Here's how the part is built. I have some questions about the finished solid (model axes, mm). Give positions to 0.01 mm unless a question says otherwise; leave off trailing zeros. Loops run counter-clockwise (first coordinate to the right, second up) from the corner with the lowest first, then second, coordinate; pieces in that order, holes last.
Q1. If we section it at A-A (z = 0): Please give me the cut outline in (x, y).
Q2. If we section it at B-B (x = -1.25): Please give me the cut outline in (y, z).
Q3. If we section it at D-D (z = 4.5): Please give me the cut outline in (x, y), plus the area to 3 significant figures.
Q4. I need wall thicknesses on line 1 (Y direction, x = -11.4, z = 0); line 2 (X direction, y = 6.25, z = -0.5); line 3 (X direction, y = 0.25, z = 9). Which ranges of each line are inside material? Lowest first, please.
Q5. We'd pull the mould along Z, two halves only. Please class faces 1 (the face through (-11.221, 9.541, 2.973)), 2 (the face through (-16.7, 0, 0)), 3 (the face through (-11.22, -9.75, 5.09)), 4 (the face through (-6.26, 0.54, 12.19)): +Z half, -Z half, draft (parallel to the pull), parting line (faces both ways), or undercut.
Q6. Will these pins go through, and if not, where does the flat tip stop? P1, Ø2, axis at x = -5, z = 2.5, coming from the -Y side; P2, Ø10, axis at x = -8, y = 8.5, coming from the +Z side; P3, Ø1.2, axis at y = 8.5, z = 5.5, coming from the -X side.
Q7. If we section it at C-C (z = -4.5): Please give me the cut outline in (x, y), plus the area to 3 significant figures.
from build123d import *

# Parameters (mm, degrees)
CUT_EXTRUDE_1_DEPTH = 3
SKETCH_4_R          = 0.75
CUT_EXTRUDE_2_DEPTH = 3
SKETCH_6_R          = 0.65
CUT_EXTRUDE_3_DEPTH = 3


with BuildPart() as part:
    # 草图1 → 旋转1 (revolve)
    with BuildSketch(Plane(origin=(0, 0, 0), x_dir=(1, 0, 0), z_dir=(0, 1, 0))):
        Polygon((0, 0), (-16.7, 0), (-16.7, 3), (-12.7, 3), (-12.7, 12.2), (0, 12.2), align=None)
    revolve(axis=Axis((-159.613189405, 0, 0), (1, 0, 0)))

    # 草图3 → 切除-拉伸1 (cut)
    with BuildSketch(Plane.ZY.offset(12.7)):
        with BuildLine():
            ThreePointArc((-8.667998766, 2.421940832), (-8.99040601, 0.415451281), (-8.854419452, -1.612220883))
            ThreePointArc((-8.854419452, -1.612220883), (-9.764043418, -2.198869939), (-10.822068219, -1.97049219))
            ThreePointArc((-10.822068219, -1.97049219), (-10.988274013, 0.507773788), (-10.594220714, 2.960149905))
            ThreePointArc((-10.594220714, 2.960149905), (-9.519642991, 3.089978996), (-8.667998766, 2.421940832))
        make_face()
        with BuildLine():
            ThreePointArc((6.43146167, 6.295736716), (4.854994369, 7.578194355), (3.030985485, 8.474262622))
            ThreePointArc((3.030985485, 8.474262622), (2.977744482, 9.555344613), (3.704537815, 10.357432094))
            ThreePointArc((3.704537815, 10.357432094), (5.933882006, 9.262237545), (7.860675374, 7.694789319))
            ThreePointArc((7.860675374, 7.694789319), (7.435821803, 6.699263167), (6.43146167, 6.295736716))
        make_face()
        with BuildLine():
            ThreePointArc((2.236537096, -8.717677547), (4.135411642, -7.993645636), (5.823433967, -6.862041739))
            ThreePointArc((5.823433967, -6.862041739), (6.786298936, -7.356474674), (7.117530404, -8.386939904))
            ThreePointArc((7.117530404, -8.386939904), (5.054392007, -9.770011333), (2.73354534, -10.654939224))
            ThreePointArc((2.73354534, -10.654939224), (2.083821188, -9.789242163), (2.236537096, -8.717677547))
        make_face()
    extrude(amount=-CUT_EXTRUDE_1_DEPTH, mode=Mode.SUBTRACT)

    # 草图4 → 切除-拉伸2 (cut)
    with BuildSketch(Plane.ZY.offset(12.7)):
        with Locations((-2.818506641, 5.448101727)):
            Circle(SKETCH_4_R)
        with Locations((-4.135411642, 7.993645636)):
            Circle(SKETCH_4_R)
        with Locations((8.99040601, -0.415451281)):
            Circle(SKETCH_4_R)
        with Locations((6.127447818, -0.283152512)):
            Circle(SKETCH_4_R)
        with Locations((-4.854994369, -7.578194355)):
            Circle(SKETCH_4_R)
        with Locations((-3.308941178, -5.164949215)):
            Circle(SKETCH_4_R)
    extrude(amount=-CUT_EXTRUDE_2_DEPTH, mode=Mode.SUBTRACT)

    # 草图6 → 切除-拉伸3 (cut)
    with BuildSketch(Plane.ZY.offset(12.7)):
        with Locations((0, 5.083503848)):
            Circle(SKETCH_6_R)
        with Locations((0, -5.083503848)):
            Circle(SKETCH_6_R)
    extrude(amount=-CUT_EXTRUDE_3_DEPTH, mode=Mode.SUBTRACT)


solid = part.part
Check sheet entries:
1. outline: (-16.7, -3) - (-12.7, -3) - (-12.7, -4.43) - (-9.7, -4.43) - (-9.7, -5.73) - (-12.7, -5.73) - (-12.7, -12.2) - (0, -12.2) - (0, 12.2) - (-12.7, 12.2) - (-12.7, 5.73) - (-9.7, 5.73) - (-9.7, 4.43) - (-12.7, 4.43) - (-12.7, 3) - (-16.7, 3) - close
2. outline: circle Ø24.4 at (0, 0)
3. outline: (-12.7, -11.34) - (0, -11.34) - (0, 11.34) - (-12.7, 11.34) - (-12.7, 10.04) - (-9.7, 10.04) - (-9.7, 7.79) - (-12.7, 7.79) - (-12.7, -7.79) - (-9.7, -7.79) - (-9.7, -10.04) - (-12.7, -10.04) - close
3. area: 275 mm2
4. line 1: y = -12.2 to -5.73, -4.43 to 4.43, 5.73 to 12.2
4. line 2: x = -12.7 to 0
4. line 3: x = -9.7 to 0
5. face 1: undercut
5. face 2: draft
5. face 3: undercut
5. face 4: parting line
6. P1: stops at y = -12.11
6. P2: stops at z = 11.69
6. P3: stops at x = -9.7
7. outline: (-12.7, -11.34) - (0, -11.34) - (0, 11.34) - (-12.7, 11.34) - (-12.7, 8.65) - (-9.7, 8.65) - (-9.7, 7.34) - (-12.7, 7.34) - (-12.7, -6.92) - (-9.7, -6.92) - (-9.7, -8.24) - (-12.7, -8.24) - close
7. area: 280 mm2
